Verification items for the finished model (mm, model axes). Round coordinates to 2 decimals unless told otherwise and drop trailing zeros. Order: outer loops, then holes, each group sorted by start corner. A loop starts at its lowest first (then second) coordinate and runs counter-clockwise, first axis right, second up. Notation, with made-up numbers: M 81,82 L 136,82 A19 cw 136,97 Z; hole C 14,67.5 d4. An arc over 180 degrees is marked long. One line per item, written item: value. Start each with the question number.
from build123d import *

# Parameters (mm, degrees)
F0_W     = 38.1
F0_H     = 107.95
F0_R     = 7.9375
F1_DEPTH = 3.175
F2_W     = 6.35
F2_H     = 3.175
F2_W_2   = 3.175
F2_H_2   = 6.35
F2_W_3   = 25.4
F2_H_3   = 44.45
F3_DEPTH = 3.175
F4_SIZE  = 4.7625


with BuildPart() as f1:
    # F0 (on Top) → F1 (new body)
    with BuildSketch(Plane.XY):
        with Locations((19.05, -53.975)):
            Rectangle(F0_W, F0_H)
        with Locations((19.05, -90.4875)):
            Circle(F0_R, mode=Mode.SUBTRACT)
        with Locations((19.05, -17.4625)):
            Circle(F0_R, mode=Mode.SUBTRACT)
    extrude(amount=F1_DEPTH)

    # F2 (on face) → F3 (cut, through all)
    with BuildSketch(Plane.XY.offset(3.175)):
        Polygon((38.1, -6.35), (38.1, 0), (34.925, 0), (34.925, -3.175), (34.925, -6.35), align=None)
        with Locations((31.75, -1.5875)):
            Rectangle(F2_W, F2_H)
        Polygon((3.175, 0), (0, 0), (0, -6.35), (3.175, -6.35), (3.175, -3.175), align=None)
        with Locations((6.35, -1.5875)):
            Rectangle(F2_W, F2_H)
        with Locations((1.5875, -15.875)):
            Rectangle(F2_W_2, F2_H_2)
        with Locations((36.5125, -15.875)):
            Rectangle(F2_W_2, F2_H_2)
        with Locations((36.5125, -28.575)):
            Rectangle(F2_W_2, F2_H_2)
        with Locations((36.5125, -41.275)):
            Rectangle(F2_W_2, F2_H_2)
        with Locations((36.5125, -53.975)):
            Rectangle(F2_W_2, F2_H_2)
        with Locations((36.5125, -66.675)):
            Rectangle(F2_W_2, F2_H_2)
        with Locations((36.5125, -79.375)):
            Rectangle(F2_W_2, F2_H_2)
        with Locations((36.5125, -92.075)):
            Rectangle(F2_W_2, F2_H_2)
        Polygon((38.1, -101.6), (34.925, -101.6), (34.925, -104.775), (34.925, -107.95), (38.1, -107.95), align=None)
        with Locations((31.75, -106.3625)):
            Rectangle(F2_W, F2_H)
        with Locations((36.5125, -117.475)):
            Rectangle(F2_W_2, F2_H_2)
        with Locations((36.5125, -130.175)):
            Rectangle(F2_W_2, F2_H_2)
        with Locations((1.5875, -28.575)):
            Rectangle(F2_W_2, F2_H_2)
        with Locations((1.5875, -41.275)):
            Rectangle(F2_W_2, F2_H_2)
        with Locations((1.5875, -53.975)):
            Rectangle(F2_W_2, F2_H_2)
        with Locations((1.5875, -66.675)):
            Rectangle(F2_W_2, F2_H_2)
        with Locations((1.5875, -79.375)):
            Rectangle(F2_W_2, F2_H_2)
        with Locations((1.5875, -92.075)):
            Rectangle(F2_W_2, F2_H_2)
        Polygon((3.175, -104.775), (3.175, -101.6), (0, -101.6), (0, -107.95), (3.175, -107.95), align=None)
        with Locations((6.35, -106.3625)):
            Rectangle(F2_W, F2_H)
        with Locations((1.5875, -117.475)):
            Rectangle(F2_W_2, F2_H_2)
        with Locations((1.5875, -130.175)):
            Rectangle(F2_W_2, F2_H_2)
        with Locations((19.05, -53.975)):
            Rectangle(F2_W_3, F2_H_3)
        with Locations((19.05, -1.5875)):
            Rectangle(F2_W, F2_H)
        with Locations((19.05, -106.3625)):
            Rectangle(F2_W, F2_H)
    extrude(amount=-F3_DEPTH, mode=Mode.SUBTRACT)

    # F4
    f4_edges = [f1.edges().sort_by_distance(p)[0] for p in [
        (31.75, -31.75, 1.5875),
        (31.75, -76.2, 1.5875),
        (6.35, -76.2, 1.5875),
        (6.35, -31.75, 1.5875),
    ]]
    chamfer(f4_edges, length=F4_SIZE)


solid = f1.part
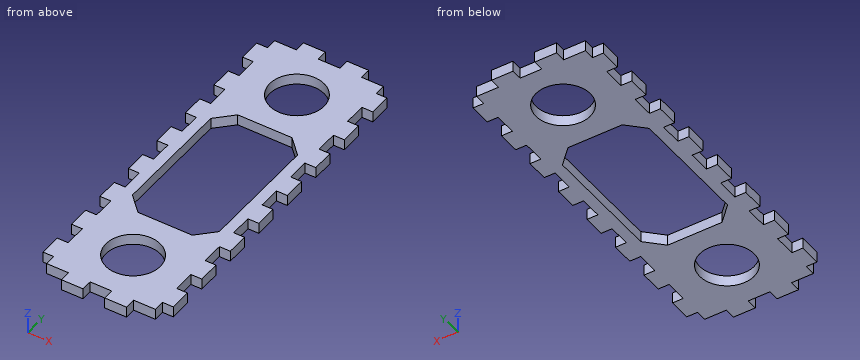
1. Section check B-B (x = 19.05). Record the cut outline in (y, z) (3 decimals).
2. Scan lines: line 1 along Y through (x, z) = (19.05, 1.15) (3 decimals); line 2 along X through (y, z) = (-68.5, 1.15) (3 decimals). Record each from-to range of solid material in increasing order.
3. Section check D-D (z = 0.8). Give the number of separate pieces and of enclosed holes in the cut face, and give its area (3 significant figures).
4. Section check A-A (y = -67). Record the cut outline in (x, z) (3 decimals).
5. Depth check by flat-ended pin: pin 1 (1 mm diameter, centred on y = -89.5, z = 1, fed in from +X) (3 decimals); pin 2 (1 mm diameter, centred on x = 36, z = 1.5, fed in from +Y); pin 3 (10 mm diameter, centred on x = 15.5, y = -96, fed in from -Z); pin 4 (1.6 mm diameter, centred on y = -54, z = 2, fed in from -X) (3 decimals). Enter the tip coordinate at first touch or a pass-through.
6. Section check C-C (y = -86). Record the cut outline in (x, z) (3 decimals), and give its area (3 significant figures).
Geometry check:
1. outline: M -104.775,0 L -98.425,0 L -98.425,3.175 L -104.775,3.175 Z; M -82.55,0 L -76.2,0 L -76.2,3.175 L -82.55,3.175 Z; M -31.75,0 L -25.4,0 L -25.4,3.175 L -31.75,3.175 Z; M -9.525,0 L -3.175,0 L -3.175,3.175 L -9.525,3.175 Z
2. line 1: y = -104.775 to -98.425, -82.55 to -76.2, -31.75 to -25.4, -9.525 to -3.175
2. line 2: x = 3.175 to 6.35, 31.75 to 34.925
3. separate pieces: 1
3. enclosed holes: 3
3. area: 2,150 mm²
4. outline: M 3.175,0 L 6.35,0 L 6.35,3.175 L 3.175,3.175 Z; M 31.75,0 L 34.925,0 L 34.925,3.175 L 31.75,3.175 Z
5. pin 1: stops at x = 34.925
5. pin 2: stops at y = -6.35
5. pin 3: stops at z = 0
5. pin 4: stops at x = 3.175
6. outline: M 0,0 L 12.503,0 L 12.503,3.175 L 0,3.175 Z; M 25.597,0 L 38.1,0 L 38.1,3.175 L 25.597,3.175 Z
6. area: 79.4 mm²
